Answer from the drawing. Dimensions are ordinates in mm from the lowest x, y and z of the part. Coordinates: 2 decimals unless noted, no trailing zeros. Write each loop counter-clockwise with the first axis right and the second up, starting at its lowest first coordinate (ties: lowest second). Pieces come first, ordered by that corner, then holes.
(1) Section A-A on z = 1.25 is taken. Write down the section's boundary in (x, y), then the cut area to 3 significant figures.
(2) Given pin 1 (2 mm diameter, centred on x = 11.5, y = 22, fed in from -Z), flat-ended and moving along its own axis, determine where the tip first touches the part or whether it passes through.
(3) Find the intervals of material crossed by probe 1 along Y at (x, z) = (25, 0.4); probe 2 along X at (y, z) = (10, 0.9); probe 3 along X at (y, z) = (42.5, 1.15), in increasing order.
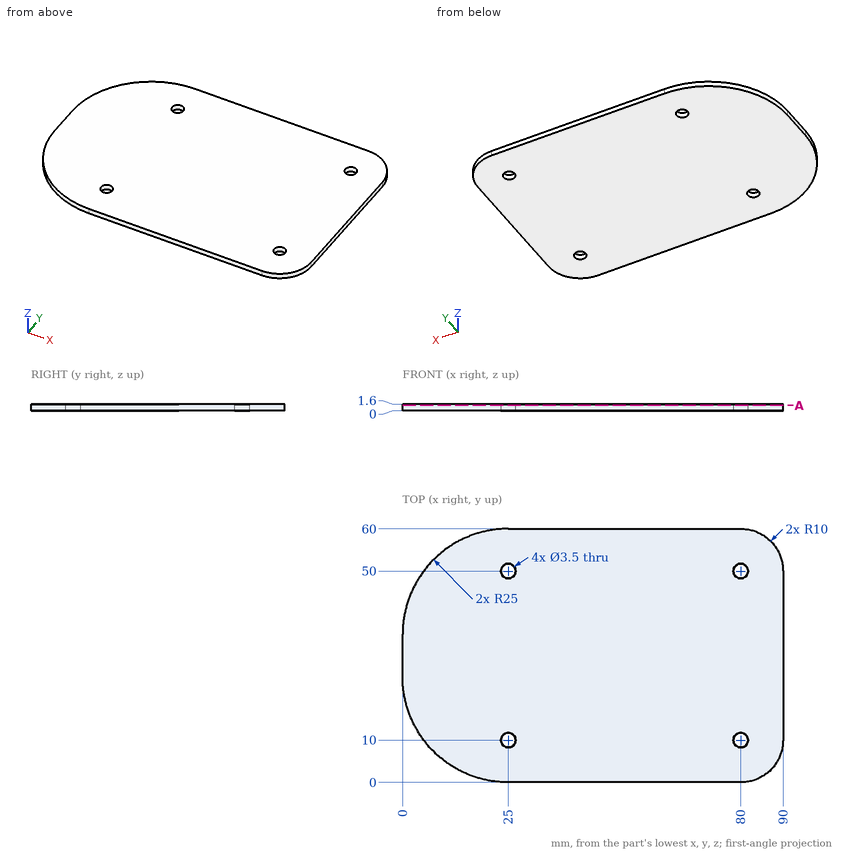
Response:
1. outline: (0, 25) arc R25 ccw to (25, 0) - (80, 0) arc R10 ccw to (90, 10) - (90, 50) arc R10 ccw to (80, 60) - (25, 60) arc R25 ccw to (0, 35) - close; hole circle Ø3.5 at (25, 10); hole circle Ø3.5 at (25, 50); hole circle Ø3.5 at (80, 10); hole circle Ø3.5 at (80, 50)
1. area: 5,050 mm2
2. pin 1: stops at z = 0
3. probe 1: y = 0 to 8.25, 11.75 to 48.25, 51.75 to 60
3. probe 2: x = 5 to 23.25, 26.75 to 78.25, 81.75 to 90
3. probe 3: x = 1.15 to 90
